```python
from build123d import *

# Parameters (mm, degrees)
SKETCH1_R           = 2.7
BOSS_EXTRUDE1_DEPTH = 6.35


with BuildPart() as part:
    # Sketch1 → Boss-Extrude1 (new body)
    with BuildSketch(Plane(origin=(6.35, 0, 0), x_dir=(0, 0, -1), z_dir=(1, 0, 0))):
        with BuildLine():
            Line((-44.45, 57.15), (-44.45, 50.8))
            Line((-44.45, 50.8), (-55.5, 50.8))
            Line((-55.5, 50.8), (-55.5, 45.8))
            Line((-55.5, 45.8), (-54.3, 45.8))
            Line((-54.3, 45.8), (-54.3, 43.3))
            Line((-54.3, 43.3), (-55.5, 43.3))
            Line((-55.5, 43.3), (-55.5, 40.8))
            Line((-55.5, 40.8), (-58.8, 40.8))
            Line((-58.8, 40.8), (-58.8, 43.3))
            Line((-58.8, 43.3), (-60, 43.3))
            Line((-60, 43.3), (-60, 45.8))
            Line((-60, 45.8), (-58.8, 45.8))
            Line((-58.8, 45.8), (-58.8, 50.8))
            Line((-58.8, 50.8), (-69.85, 50.8))
            Line((-69.85, 50.8), (-69.85, 57.15))
            Line((-69.85, 57.15), (-152.4, 57.15))
            Line((-152.4, 57.15), (-152.4, 50.8))
            Line((-152.4, 50.8), (-163.45, 50.8))
            Line((-163.45, 50.8), (-163.45, 45.8))
            Line((-163.45, 45.8), (-162.25, 45.8))
            Line((-162.25, 45.8), (-162.25, 43.3))
            Line((-162.25, 43.3), (-163.45, 43.3))
            Line((-163.45, 43.3), (-163.45, 40.8))
            Line((-163.45, 40.8), (-166.75, 40.8))
            Line((-166.75, 40.8), (-166.75, 43.3))
            Line((-166.75, 43.3), (-167.95, 43.3))
            Line((-167.95, 43.3), (-167.95, 45.8))
            Line((-167.95, 45.8), (-166.75, 45.8))
            Line((-166.75, 45.8), (-166.75, 50.8))
            Line((-166.75, 50.8), (-177.8, 50.8))
            Line((-177.8, 50.8), (-177.8, 57.15))
            Line((-177.8, 57.15), (-215.9, 57.15))
            Line((-215.9, 57.15), (-215.9, 47.6875))
            Line((-215.9, 47.6875), (-210.9, 47.6875))
            Line((-210.9, 47.6875), (-210.9, 48.8875))
            Line((-210.9, 48.8875), (-208.4, 48.8875))
            Line((-208.4, 48.8875), (-208.4, 47.6875))
            Line((-208.4, 47.6875), (-205.9, 47.6875))
            Line((-205.9, 47.6875), (-205.9, 44.3875))
            Line((-205.9, 44.3875), (-208.4, 44.3875))
            Line((-208.4, 44.3875), (-208.4, 43.1875))
            Line((-208.4, 43.1875), (-210.9, 43.1875))
            Line((-210.9, 43.1875), (-210.9, 44.3875))
            Line((-210.9, 44.3875), (-215.9, 44.3875))
            Line((-215.9, 44.3875), (-215.9, 34.925))
            Line((-215.9, 34.925), (-222.25, 34.925))
            Line((-222.25, 34.925), (-222.25, 22.225))
            Line((-222.25, 22.225), (-215.9, 22.225))
            Line((-215.9, 22.225), (-215.9, 12.7625))
            Line((-215.9, 12.7625), (-210.9, 12.7625))
            Line((-210.9, 12.7625), (-210.9, 13.9625))
            Line((-210.9, 13.9625), (-208.4, 13.9625))
            Line((-208.4, 13.9625), (-208.4, 12.7625))
            Line((-208.4, 12.7625), (-205.9, 12.7625))
            Line((-205.9, 12.7625), (-205.9, 9.4625))
            Line((-205.9, 9.4625), (-208.4, 9.4625))
            Line((-208.4, 9.4625), (-208.4, 8.2625))
            Line((-208.4, 8.2625), (-210.9, 8.2625))
            Line((-210.9, 8.2625), (-210.9, 9.4625))
            Line((-210.9, 9.4625), (-215.9, 9.4625))
            Line((-215.9, 9.4625), (-215.9, 0))
            Line((-215.9, 0), (-160.59896879, 0))
            ThreePointArc((-160.59896879, 0), (-158.861506462, 0.306361486), (-157.333607733, 1.188494229))
            Line((-157.333607733, 1.188494229), (-139.588074729, 16.078764428))
            ThreePointArc((-139.588074729, 16.078764428), (-135.768327906, 18.284096284), (-131.424672086, 19.05))
            Line((-131.424672086, 19.05), (131.424672086, 19.05))
            ThreePointArc((131.424672086, 19.05), (135.768327906, 18.284096284), (139.588074729, 16.078764428))
            Line((139.588074729, 16.078764428), (157.333607733, 1.188494229))
            ThreePointArc((157.333607733, 1.188494229), (158.861506462, 0.306361486), (160.59896879, 0))
            Line((160.59896879, 0), (215.9, 0))
            Line((215.9, 0), (215.9, 9.4625))
            Line((215.9, 9.4625), (210.9, 9.4625))
            Line((210.9, 9.4625), (210.9, 8.2625))
            Line((210.9, 8.2625), (208.4, 8.2625))
            Line((208.4, 8.2625), (208.4, 9.4625))
            Line((208.4, 9.4625), (205.9, 9.4625))
            Line((205.9, 9.4625), (205.9, 12.7625))
            Line((205.9, 12.7625), (208.4, 12.7625))
            Line((208.4, 12.7625), (208.4, 13.9625))
            Line((208.4, 13.9625), (210.9, 13.9625))
            Line((210.9, 13.9625), (210.9, 12.7625))
            Line((210.9, 12.7625), (215.9, 12.7625))
            Line((215.9, 12.7625), (215.9, 22.225))
            Line((215.9, 22.225), (222.25, 22.225))
            Line((222.25, 22.225), (222.25, 34.925))
            Line((222.25, 34.925), (215.9, 34.925))
            Line((215.9, 34.925), (215.9, 44.3875))
            Line((215.9, 44.3875), (210.9, 44.3875))
            Line((210.9, 44.3875), (210.9, 43.1875))
            Line((210.9, 43.1875), (208.4, 43.1875))
            Line((208.4, 43.1875), (208.4, 44.3875))
            Line((208.4, 44.3875), (205.9, 44.3875))
            Line((205.9, 44.3875), (205.9, 47.6875))
            Line((205.9, 47.6875), (208.4, 47.6875))
            Line((208.4, 47.6875), (208.4, 48.8875))
            Line((208.4, 48.8875), (210.9, 48.8875))
            Line((210.9, 48.8875), (210.9, 47.6875))
            Line((210.9, 47.6875), (215.9, 47.6875))
            Line((215.9, 47.6875), (215.9, 57.15))
            Line((215.9, 57.15), (177.8, 57.15))
            Line((177.8, 57.15), (177.8, 50.8))
            Line((177.8, 50.8), (163.575, 50.8))
            Line((163.575, 50.8), (163.575, 45.8))
            Line((163.575, 45.8), (164.775, 45.8))
            Line((164.775, 45.8), (164.775, 43.3))
            Line((164.775, 43.3), (163.575, 43.3))
            Line((163.575, 43.3), (163.575, 40.8))
            Line((163.575, 40.8), (160.275, 40.8))
            Line((160.275, 40.8), (160.275, 43.3))
            Line((160.275, 43.3), (159.075, 43.3))
            Line((159.075, 43.3), (159.075, 45.8))
            Line((159.075, 45.8), (160.275, 45.8))
            Line((160.275, 45.8), (160.275, 50.8))
            Line((160.275, 50.8), (146.05, 50.8))
            Line((146.05, 50.8), (146.05, 57.15))
            Line((146.05, 57.15), (63.5, 57.15))
            Line((63.5, 57.15), (63.5, 50.8))
            Line((63.5, 50.8), (52.45, 50.8))
            Line((52.45, 50.8), (52.45, 45.8))
            Line((52.45, 45.8), (53.65, 45.8))
            Line((53.65, 45.8), (53.65, 43.3))
            Line((53.65, 43.3), (52.45, 43.3))
            Line((52.45, 43.3), (52.45, 40.8))
            Line((52.45, 40.8), (49.15, 40.8))
            Line((49.15, 40.8), (49.15, 43.3))
            Line((49.15, 43.3), (47.95, 43.3))
            Line((47.95, 43.3), (47.95, 45.8))
            Line((47.95, 45.8), (49.15, 45.8))
            Line((49.15, 45.8), (49.15, 50.8))
            Line((49.15, 50.8), (38.1, 50.8))
            Line((38.1, 50.8), (38.1, 57.15))
            Line((38.1, 57.15), (-44.45, 57.15))
        make_face()
        with Locations(Location((79.988301448, 33.74898, 0), (0, 0, 180))):
            Circle(SKETCH1_R, mode=Mode.SUBTRACT)
        with Locations(Location((130.788301448, 33.74898, 0), (0, 0, 180))):
            Circle(SKETCH1_R, mode=Mode.SUBTRACT)
        with Locations(Location((29.188301448, 33.74898, 0), (0, 0, 180))):
            Circle(SKETCH1_R, mode=Mode.SUBTRACT)
        with Locations(Location((181.588301448, 33.74898, 0), (0, 0, 180))):
            Circle(SKETCH1_R, mode=Mode.SUBTRACT)
    extrude(amount=-BOSS_EXTRUDE1_DEPTH)


solid = part.part
```
The model under review builds one solid part; all positions refer to its coordinate system, in mm. A direction names the side the tool comes from. Round coordinates to 2 decimals unless told otherwise and drop trailing zeros. Loops run counter-clockwise (first coordinate to the right, second up) from the corner with the lowest first, then second, coordinate; pieces in that order, holes last. Notation, with made-up numbers: (-33, -1) -> (-2, -1) arc R28 cw to (-2, 19) -> close; hole circle Ø9 at (61.5, 16.25). An arc over 180 degrees is marked (long way). Answer in a Markdown table with one row per item.
1) Wall thickness on line 1 along Z through (x, y) = (1.5, 47) (3 decimals); line 2 along Z through (x, y) = (3.75, 53); line 3 along Z through (x, y) = (3.75, 13): over which ranges is each line inside the solid? List them lowest first.
Taken from the geometry:
| item | result |
|---|---|
| line 1 | z = -205.9 to -163.575, -160.275 to -52.45, -49.15 to 55.5, 58.8 to 163.45, 166.75 to 205.9 |
| line 2 | z = -215.9 to -177.8, -146.05 to -63.5, -38.1 to 44.45, 69.85 to 152.4, 177.8 to 215.9 |
| line 3 | z = -215.9 to -210.9, -208.4 to -143.26, 143.26 to 208.4, 210.9 to 215.9 |
2) Consider section C-C, the plane z = 145. Write out the cut boundary in (x, y).
Taken from the geometry:
| item | result |
|---|---|
| outline | (0, 11.54) -> (6.35, 11.54) -> (6.35, 57.15) -> (0, 57.15) -> close |
3) Consider section A-A, the plane z = 24. Write out the cut boundary in (x, y), plus the area to 3 significant figures.
Taken from the geometry:
| item | result |
|---|---|
| outline | (0, 19.05) -> (6.35, 19.05) -> (6.35, 57.15) -> (0, 57.15) -> close |
| area | 242 mm² |
4) Consider section B-B, the plane x = 4.5. Count the separate pieces of the cut face and the enclosed holes in it, plus the area to 3 significant figures.
Taken from the geometry:
| item | result |
|---|---|
| separate pieces | 1 |
| enclosed holes | 4 |
| area | 18,100 mm² |
5) Tool access review of faces 1 (the flat face through (0, 35, 3)), 2 (the flat face through (3.219, 8.738, -148.337)): name each direction out of +Z, -Z, +X, -X, +Y, -Y from which nothing blocks a thin tool from reaching the whole face with its end or side.
Taken from the geometry:
| item | result |
|---|---|
| face 1 | +Z, -Z, -X, +Y, -Y |
| face 2 | +X, -X, -Y |
6) For pin 1 Ø2 at (x, y) = (4.5, 41.5) entering from -Z; pin 2 Ø0.8 at (x, y) = (4.5, 42) entering from +Z, all flat-tipped, find the tip position at first contact; note any pin that passes through.
Taken from the geometry:
| item | result |
|---|---|
| pin 1 | stops at z = -215.9 |
| pin 2 | stops at z = 215.9 |
7) Draft analysis for pull direction Z (two halves, no side actions). For faces 3 (the flat face through (3.219, 8.529, 148.585)), 4 (the flat face through (6.35, 35, 3)), state which applies: pulls with the +Z half, pulls with the -Z half, needs draft (parallel to the pull), parting line crosses it, or undercut.
Taken from the geometry:
| item | result |
|---|---|
| face 3 | undercut |
| face 4 | needs draft |
